Geometry check sheet. Reference: drawing and pictorial views, mm from the part's lowest x, y, z. A direction names the side the tool comes from. Round coordinates to 2 decimals unless told otherwise and drop trailing zeros. Loops run counter-clockwise (first coordinate to the right, second up) from the corner with the lowest first, then second, coordinate; pieces in that order, holes last. Notation, with made-up numbers: (54, -38) - (89, -38) arc R36 ccw to (89, 1) - close; hole circle Ø4 at (-27, 70). An arc over 180 degrees is marked (long way). Put each result on its own line as item: value. Start each with the question number.
Item 1: Gauge pin test, flat ends, axial feed: pin 1 Ø22 at (y, z) = (42.5, 37) entering from -X; pin 2 Ø22 at (x, y) = (168.5, 81.5) entering from -Z; pin 3 Ø16 at (x, y) = (168, 57.5) entering from +Z. Record the tip position at first contact, or that the pin passes through.
Item 2: Tool access check on the marked faces 1, 2 and 3. Record the directions out of +Z, -Z, +X, -X, +Y, -Y that give a thin tool (end or side, any length) a straight path to the whole face; none if there is none.
Item 3: Section check C-C, the plane z = 40. Record the cut outline in (x, y).
Item 4: Section check A-A, the plane x = 168. Record the cut outline in (y, z), and give its area (3 significant figures).
Item 5: Material ranges on line 1 along X through (y, z) = (199, 17.5); line 2 along Y through (x, z) = (104.5, 41); line 3 along X through (y, z) = (360, 11.5), recorded low to high.
Item 6: Section check D-D, the plane y = 35.5. Record the cut outline in (x, z), and give its area (3 significant figures).
Item 7: Section check B-B, the plane y = 492.5. Record the cut outline in (x, z).
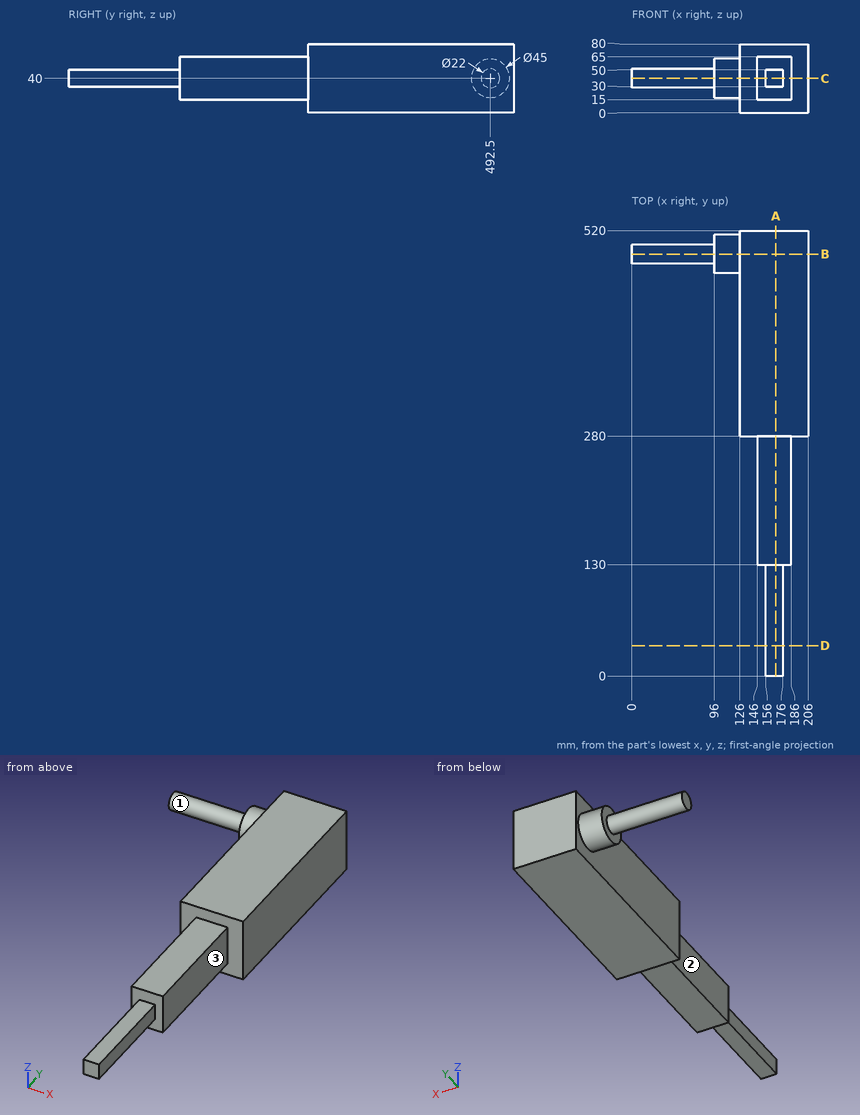
Check result:
1. pin 1: x = 156
1. pin 2: z = 30
1. pin 3: z = 50
2. face 1: -X
2. face 2: +Z, -Z, -X, -Y
2. face 3: +Z, -Z, +X, -Y
3. outline: (0, 481.5) - (96, 481.5) - (96, 470) - (126, 470) - (126, 280) - (146, 280) - (146, 130) - (156, 130) - (156, 0) - (176, 0) - (176, 130) - (186, 130) - (186, 280) - (206, 280) - (206, 520) - (126, 520) - (126, 515) - (96, 515) - (96, 503.5) - (0, 503.5) - close
4. outline: (0, 30) - (130, 30) - (130, 15) - (280, 15) - (280, 0) - (520, 0) - (520, 80) - (280, 80) - (280, 65) - (130, 65) - (130, 50) - (0, 50) - close
4. area: 29,300 mm²
5. line 1: 146 to 186
5. line 2: 470.02 to 514.98
5. line 3: 126 to 206
6. outline: (156, 30) - (176, 30) - (176, 50) - (156, 50) - close
6. area: 400 mm²
7. outline: (0, 29) - (96, 29) - (96, 17.5) - (126, 17.5) - (126, 0) - (206, 0) - (206, 80) - (126, 80) - (126, 62.5) - (96, 62.5) - (96, 51) - (0, 51) - close
